from build123d import *

# Parameters (mm, degrees)
SKETCH1_W                = 138.816596539
SKETCH1_H                = 51.704152624
BOSS_EXTRUDE1_DEPTH      = 4
SKETCH2_R                = 19.5
CUT_EXTRUDE1_DEPTH       = 4
SKETCH3_W                = 39
SKETCH3_H                = 25.518890855
CUT_EXTRUDE2_DEPTH       = 4
SKETCH4_W                = 138.816596539
SKETCH4_H                = 5.527763413
CUT_EXTRUDE3_DEPTH       = 4
CUT_EXTRUDE4_DEPTH       = 4
BOSS_EXTRUDE2_DEPTH      = 7
CUT_EXTRUDE6_DEPTH       = 10
CUT_EXTRUDE6_DEPTH_BACK  = 1
SKETCH8_W                = 41.210335228
SKETCH8_H                = 18.724016431
FILLET1_R                = 4
SKETCH9_W                = 159.262648619
SKETCH9_H                = 8.218574615
CUT_EXTRUDE7_DEPTH       = 13
SKETCH10_W               = 138.816596539
SKETCH10_H               = 3.381053597
BOSS_EXTRUDE3_DEPTH      = 112
CUT_EXTRUDE8_DEPTH       = 6
BOSS_EXTRUDE4_DEPTH      = 5
BOSS_EXTRUDE5_DEPTH      = 5
BOSS_EXTRUDE6_DEPTH      = 3
BOSS_EXTRUDE6_DEPTH_BACK = 3


with BuildPart() as part:
    # Sketch1 → Boss-Extrude1 (new body)
    with BuildSketch(Plane(origin=(0, 0, 0), x_dir=(1, 0, 0), z_dir=(0, 1, 0))):
        with Locations((69.40829827, 25.852076312)):
            Rectangle(SKETCH1_W, SKETCH1_H)
    extrude(amount=BOSS_EXTRUDE1_DEPTH)

    # Sketch2 → Cut-Extrude1 (cut)
    with BuildSketch(Plane(origin=(0, 4, 0), x_dir=(1, 0, 0), z_dir=(0, 1, 0))):
        with Locations(Location((32.40871363, 26.185261769, 0), (0, 0, 270))):
            Circle(SKETCH2_R)
        with Locations(Location((105.33778471, 26.185261769, 0), (0, 0, 270))):
            Circle(SKETCH2_R)
    extrude(amount=-CUT_EXTRUDE1_DEPTH, mode=Mode.SUBTRACT)

    # Sketch3 → Cut-Extrude2 (cut)
    with BuildSketch(Plane(origin=(0, 4, 0), x_dir=(1, 0, 0), z_dir=(0, 1, 0))):
        with Locations((32.40871363, 38.944707197)):
            Rectangle(SKETCH3_W, SKETCH3_H)
        with Locations((105.33778471, 38.944707197)):
            Rectangle(SKETCH3_W, SKETCH3_H)
    extrude(amount=-CUT_EXTRUDE2_DEPTH, mode=Mode.SUBTRACT)

    # Sketch4 → Cut-Extrude3 (cut)
    with BuildSketch(Plane(origin=(0, 4, 0), x_dir=(1, 0, 0), z_dir=(0, 1, 0))):
        with Locations((69.40829827, 48.940270918)):
            Rectangle(SKETCH4_W, SKETCH4_H)
    extrude(amount=-CUT_EXTRUDE3_DEPTH, mode=Mode.SUBTRACT)

    # Sketch5 → Cut-Extrude4 (cut)
    with BuildSketch(Plane(origin=(0, 4, 0), x_dir=(1, 0, 0), z_dir=(0, 1, 0))):
        Polygon((51.928250722, 38.363055383), (49.904010148, 40.387295957), (49.904010148, 49.123987915), (88.976343822, 49.123987915), (88.23099636, 41.297839561), (87.953832157, 40.819568311), (85.857321802, 38.348253507), (84.416556547, 36.649914887), (53.389948025, 36.649914887), align=None)
    extrude(amount=-CUT_EXTRUDE4_DEPTH, mode=Mode.SUBTRACT)

    # Sketch6 → Boss-Extrude2 (add)
    with BuildSketch(Plane(origin=(0, 4, 0), x_dir=(1, 0, 0), z_dir=(0, 1, 0))):
        with BuildLine():
            Line((53.27008085, 36.472479648), (84.296689371, 36.472479648))
            Line((84.296689371, 36.472479648), (73.621100147, 23.890682137))
            ThreePointArc((73.621100147, 23.890682137), (68.737776852, 21.92042398), (63.891562932, 23.980272094))
            Line((63.891562932, 23.980272094), (53.27008085, 36.472479648))
        make_face()
    extrude(amount=BOSS_EXTRUDE2_DEPTH)

    # Sketch8 → Cut-Extrude6 (cut, two sides: drawn at the far end of the back side and taken through both)
    with BuildSketch(Plane(origin=(0, 0, -36.649914887), x_dir=(-1, 0, 0), z_dir=(0, 0, -1)).offset(-CUT_EXTRUDE6_DEPTH_BACK)):
        with Locations((-66.917709276, 5.20508787)):
            Rectangle(SKETCH8_W, SKETCH8_H)
    extrude(amount=CUT_EXTRUDE6_DEPTH + CUT_EXTRUDE6_DEPTH_BACK, mode=Mode.SUBTRACT)

    # Fillet1
    fillet1_edges = [part.edges().sort_by_distance(p)[0] for p in [
        (85.83778471, 2, -35.649914887),
        (51.90871363, 2, -35.649914887),
    ]]
    fillet(fillet1_edges, radius=FILLET1_R)

    # Sketch9 → Cut-Extrude7 (cut)
    with BuildSketch(Plane(origin=(0, 4, 0), x_dir=(1, 0, 0), z_dir=(0, 1, 0))):
        with Locations((71.074225557, -1.789652878)):
            Rectangle(SKETCH9_W, SKETCH9_H)
    extrude(amount=-CUT_EXTRUDE7_DEPTH, mode=Mode.SUBTRACT)

    # Sketch10 → Boss-Extrude3 (add)
    with BuildSketch(Plane(origin=(0, 0, 0), x_dir=(-1, 0, 0), z_dir=(0, -1, 0))):
        with Locations((-69.40829827, 4.010161229)):
            Rectangle(SKETCH10_W, SKETCH10_H)
    extrude(amount=BOSS_EXTRUDE3_DEPTH)

    # Sketch11 → Cut-Extrude8 (cut)
    with BuildSketch(Plane(origin=(0, 0, -5.700688027), x_dir=(-1, 0, 0), z_dir=(0, 0, -1))):
        with BuildLine():
            Line((-51.833864247, -74.608061362), (-51.833864247, -112))
            Line((-51.833864247, -112), (-86.982732292, -112))
            Line((-86.982732292, -112), (-86.982732292, -74.608061362))
            ThreePointArc((-86.982732292, -74.608061362), (-69.40829827, -57.033627339), (-51.833864247, -74.608061362))
        make_face()
    extrude(amount=-CUT_EXTRUDE8_DEPTH, mode=Mode.SUBTRACT)

    # Sketch12 → Boss-Extrude4 (add)
    with BuildSketch(Plane.ZY):
        Polygon((-46.176389211, 0), (-5.700688027, 0), (-5.700688027, -56), align=None)
    extrude(amount=-BOSS_EXTRUDE4_DEPTH)

    # Sketch13 → Boss-Extrude5 (add)
    with BuildSketch(Plane(origin=(138.816596539, 0, 0), x_dir=(0, 0, -1), z_dir=(1, 0, 0))):
        Polygon((5.700688027, 0), (46.176389211, 0), (5.700688027, -56), align=None)
    extrude(amount=-BOSS_EXTRUDE5_DEPTH)

    # Sketch14 → Boss-Extrude6 (add, two sides: drawn at the far end of the back side and taken through both)
    with BuildSketch(Plane(origin=(69, 0, 0), x_dir=(0, 0, -1), z_dir=(1, 0, 0)).offset(-BOSS_EXTRUDE6_DEPTH_BACK)):
        Polygon((5.700688027, 0), (35.649914887, 0), (5.700688027, -41.436137117), align=None)
    extrude(amount=BOSS_EXTRUDE6_DEPTH + BOSS_EXTRUDE6_DEPTH_BACK)


solid = part.part
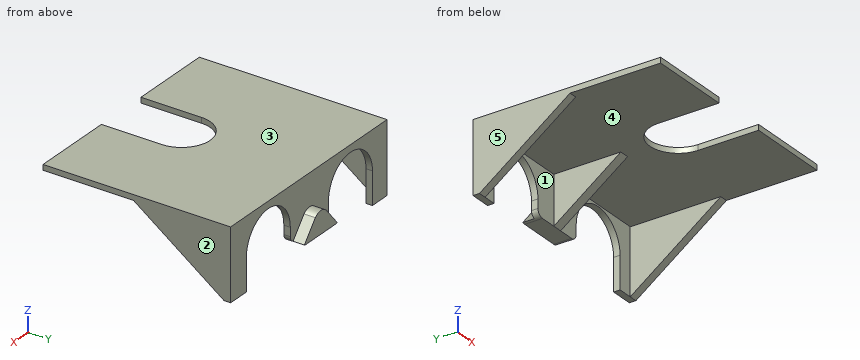
Input: part model. Units: mm. Frame: model coordinates. Face numbers are marked on the shaded views. A direction names the side the tool comes from. Give positions to 0.01 mm unless a question says otherwise; leave off trailing zeros. Order: outer loops, then holes, each group sorted by start corner. A loop starts at its lowest first (then second) coordinate and runs counter-clockwise, first axis right, second up. Notation, with made-up numbers: (87, 89) - (127, 89) arc R29 ccw to (127, 118) - close; hole circle Ø9 at (28, 63). An arc over 180 degrees is marked (long way). Answer as a JSON object with one key per item and string values. Group by question number.
Q1. Cut plane D-D, the plane y = -28.5. Output: boundary loops of the cut face in (x, z), then the cut area to 3 significant figures.
Q2. Set-up query: the marked faces 4 and 5. Return all of +Z, -Z, +X, -X, +Y, -Y with unobstructed straight access to the full face (end or side cutting, diameter ignored); none if empty.
Q3. Cut plane C-C, the plane z = -9. Output: boundary loops of the cut face in (x, y).
Q4. Cut plane A-A, the plane y = -100.5. Output: boundary loops of the cut face in (x, z), then the cut area to 3 significant figures.
Q5. Line query: probe 1 along X at (y, z) = (-20, -11); probe 2 along X at (y, z) = (-33, -16.5); probe 3 along Z at (x, y) = (45, -36.5). Output: solid intervals per line, ascending.
Q6. First-contact query: pin 1 Ø4 at (y, z) = (-21.5, -31.5) entering from +X; pin 2 Ø1.5 at (x, z) = (88, -16) entering from +Y; pin 3 Ø12 at (x, y) = (112.5, -35.5) entering from -Z; pin 4 Ø12 at (x, y) = (70, 7.5) entering from -Z. Flat tips, straight axial feed; report the tip coordinate or a pass-through.
Q7. Mould query, pull axis X, two halves, no side actions, for the marked faces 1, 2 and 3. Classes: pulls with the +X half, pulls with the -X half, needs draft (parallel to the pull), parting line crosses it, or undercut.
Q8. Cut plane B-B, the plane z = -41. Output: boundary loops of the cut face in (x, y), then the cut area to 3 significant figures.
Results:
{
 "1": {"outline": "(0, -25.58) - (5, -25.58) - (5, -5.7) - (66, -5.7) - (66, -15.05) - (72, -15.05) - (72, -5.7) - (133.82, -5.7) - (133.82, -25.58) - (138.82, -25.58) - (138.82, -2.32) - (0, -2.32) - close", "area": "724 mm^2"},
 "2": {"face 4": "-Z, -Y", "face 5": "+Z, -Z, -X, +Y, -Y"},
 "3": {"outline": "(0, -51.44) - (5, -51.44) - (5, 0) - (23.19, 0) - (23.19, 4) - (0, 4) - close; (41.62, 0) - (66, 0) - (66, -36.87) - (72, -36.87) - (72, 0) - (96.12, 0) - (96.12, 4) - (41.62, 4) - close; (114.55, 0) - (133.82, 0) - (133.82, -51.44) - (138.82, -51.44) - (138.82, 4) - (114.55, 4) - close"},
 "4": {"outline": "(0, -5.7) - (51.83, -5.7) - (51.83, -2.32) - (0, -2.32) - close; (86.98, -5.7) - (138.82, -5.7) - (138.82, -2.32) - (86.98, -2.32) - close", "area": "351 mm^2"},
 "5": {"probe 1": "0 to 5, 66 to 72, 133.82 to 138.82", "probe 2": "0 to 5, 133.82 to 138.82", "probe 3": "-5.7 to -2.32"},
 "6": {"pin 1": "x = 138.82", "pin 2": "y = 4", "pin 3": "z = -5.7", "pin 4": "z = -35.65"},
 "7": {"face 1": "undercut", "face 2": "pulls with the +X half", "face 3": "needs draft"},
 "8": {"outline": "(0, -7.16) - (5, -7.16) - (5, 0) - (12.91, 0) - (12.91, 4) - (0, 4) - close; (124.84, 0) - (133.82, 0) - (133.82, -7.16) - (138.82, -7.16) - (138.82, 4) - (124.84, 4) - close", "area": "179 mm^2"}
}
